Autodesk Inventor part; units mm, degrees
ref_plane "part2_to_part1_XY" through (0, 0, 0) normal (1, 0, 0) x (0, 0, -1)
ref_plane "part2_to_part1_YZ" through (0, 0, 0) normal (0, 0, -1) x (0, 1, 0)
ref_plane "part2_to_part1_ZX" through (0, 0, 0) normal (0, 1, 0) x (1, 0, 0)
sketch "Sketch_1" plane through (0, 0, 0) normal (0, 0, 1) x (1, 0, 0)
  line L0 (10, 0) -> (0, 0)
  line L1 (1, 5) -> (10, 5)
  line L2 (10, 5) -> (10, 12)
  line L3 (10, 12) -> (9.5, 12.5)
  line L4 (9.5, 12.5) -> (1, 12.5)
  line L5 (1, 12.5) -> (1, 5)
revolve "Revolution1" add sketch "Sketch_1" angle 180 mid plane about axis through (10, 0, 0) along (-1, 0, 0)
sketch "Sketch_2" plane through (0, 0, 0) normal (0, 0, 1) x (1, 0, 0)
  line L0 (0, 0.5) -> (0, 0)
  line L1 (0, 0) -> (20, 0)
  line L2 (20, 0) -> (20, 0.5)
  line L3 (20, 0.5) -> (0, 0.5)
extrude "Extrusion1" cut sketch "Sketch_2" along normal mid plane 50
sketch "Sketch_3" plane through (0, 0, 9) normal (0, 0, 1) x (1, 0, 0)
  line L0 (5.5, 12.5) -> (5.5, 0)
  line L1 (5.5, 0) -> (3.25, 0)
  line L2 (3.25, 0) -> (3.25, 4.5)
  line L3 (3.25, 4.5) -> (1.5, 4.5)
  line L4 (1.5, 4.5) -> (1.5, 12.5)
  line L5 (1.5, 12.5) -> (5.5, 12.5)
  line L6 (5.5, 12.5) -> (5.5, 0)
revolve "Revolution2" cut sketch "Sketch_3" angle 360 about axis through (5.5, 12.5, 9) along (0, 1, 0)
sketch "Sketch_4" plane through (0, 0, -9) normal (0, 0, 1) x (1, 0, 0)
  line L0 (5.5, 12.5) -> (5.5, 0)
  line L1 (5.5, 0) -> (3.25, 0)
  line L2 (3.25, 0) -> (3.25, 4.5)
  line L3 (3.25, 4.5) -> (1.5, 4.5)
  line L4 (1.5, 4.5) -> (1.5, 12.5)
  line L5 (1.5, 12.5) -> (5.5, 12.5)
  line L6 (5.5, 12.5) -> (5.5, 0)
revolve "Revolution3" cut sketch "Sketch_4" angle 360 about axis through (5.5, 12.5, -9) along (0, 1, 0)
sketch "Sketch_5" plane through (0, 0, 9) normal (0, 0, 1) x (1, 0, 0)
  line L0 (0, 17) -> (0, 4.5)
  line L1 (0, 4.5) -> (20, 4.5)
  line L2 (20, 4.5) -> (20, 17)
  line L3 (20, 17) -> (0, 17)
extrude "Extrusion2" cut sketch "Sketch_5" along normal blind 25
sketch "Sketch_6" plane through (0, 0, -9) normal (0, 0, 1) x (1, 0, 0)
  line L0 (0, 17) -> (0, 4.5)
  line L1 (0, 4.5) -> (20, 4.5)
  line L2 (20, 4.5) -> (20, 17)
  line L3 (20, 17) -> (0, 17)
extrude "Extrusion3" cut sketch "Sketch_6" against normal blind 25
ref_plane "part2_to_part1_XY" through (0, 0, 0) normal (1, 0, 0) x (0, 0, -1)
ref_plane "part2_to_part1_YZ" through (0, 0, 0) normal (0, 0, -1) x (0, 1, 0)
ref_plane "part2_to_part1_ZX" through (0, 0, 0) normal (0, 1, 0) x (1, 0, 0)
ref_plane "part2_to_screw1_XY" through (5.5, 4.5, 9) normal (0, 1, 0) x (1, 0, 0)
ref_plane "part2_to_screw1_YZ" through (5.5, 4.5, 9) normal (1, 0, 0) x (0, 0, -1)
ref_plane "part2_to_screw1_ZX" through (5.5, 4.5, 9) normal (0, 0, -1) x (0, 1, 0)
ref_plane "part2_to_screw2_XY" through (5.5, 4.5, -9) normal (0, 1, 0) x (1, 0, 0)
ref_plane "part2_to_screw2_YZ" through (5.5, 4.5, -9) normal (1, 0, 0) x (0, 0, -1)
ref_plane "part2_to_screw2_ZX" through (5.5, 4.5, -9) normal (0, 0, -1) x (0, 1, 0)
properties part number "MBRAC45-2-10p2"
CAD build for the part. Positions are in the model's coordinates, mm. A direction names the side the tool comes from. Coordinates: 2 decimals unless noted, no trailing zeros. Loops run counter-clockwise (first coordinate to the right, second up) from the corner with the lowest first, then second, coordinate; pieces in that order, holes last. Notation, with made-up numbers: (2, 70) - (14, 70) arc R18 cw to (14, 74) - close; hole circle Ø6 at (67.25, 37). An arc over 180 degrees is marked (long way). Use CSV: the item, a comma, the result in double quotes. Start each with the question number.
Q1. Cut at A-A, the plane x = 5.5. List the corners of the cut face in (y, z).
Q2. Probe probe 1 along X at (y, z) = (3.4, -9); probe 2 along Z at (x, y) = (5.5, 3.2); probe 3 along Z at (x, y) = (4.25, 1.25). List the from-to ranges inside material, lowest first. Write a range as from..to.
Q3. Cut at C-C, the plane y = 1.75. State how many separate pieces and enclosed holes the cut face has, then the cut area to 3 significant figures.
Q4. 3-axis set-ups, long thin cutter, end or side, ignore diameter. For faces 1 (the flat face through (7, 0.5, 7)), 2 (the flat face through (4, 4.5, 7)), 3 (the cylindrical face through (5.4, 7.3, -5)): which of +Z, -Z, +X, -X, +Y, -Y reach the whole face in a straight line?
Q5. Drop flat-ended pins along their axis: P1, Ø3.5, axis at x = 3.5, z = -9.5, coming from the +Y side; P2, Ø0.6, axis at x = 1, y = 6, coming from the +Z side; P3, Ø1, axis at x = 5, y = 3.5, coming from the +Z side. Give the stop position or say it passes through.
Q6. Cut at D-D, the plane x = 3.5. List the corners of the cut face in (y, z).
Q7. Cut at B-B, the plane y = 6.25. List the corners of the cut face in (x, z).
Q8. Two-plate mould, pull along X, no slides. Class faces 4 (the flat face through (4, 4.5, -7)), 5 (the flat face through (1, 7, 0)), 6 (the flat face through (8, 0.5, -8)), 7 (the cylindrical face through (4.29, 2.528, 10.897)): +X half, -X half, draft (parallel to the pull), parting line (faces both ways), or undercut.
Here are the results:
1,outline,"(0.5, -12.49) arc R12.5 ccw to (4.5, -11.66) - (4.5, -11.25) - (0.5, -11.25) - close; (0.5, -6.75) - (4.5, -6.75) - (4.5, -5) - (11.46, -5) arc R12.5 ccw to (11.46, 5) - (4.5, 5) - (4.5, 6.75) - (0.5, 6.75) - (0.5, 4.97) arc R5 cw to (0.5, -4.97) - close; (0.5, 11.25) - (4.5, 11.25) - (4.5, 11.66) arc R12.5 ccw to (0.5, 12.49) - close"
2,probe 1,"1..3.25, 7.75..10"
2,probe 2,"-12.08..-11.25, -6.75..-3.84, 3.84..6.75, 11.25..12.08"
2,probe 3,"-12.44..-10.87, -7.13..-4.84, 4.84..7.13, 10.87..12.44"
3,separate pieces,"2"
3,enclosed holes,"2"
3,area,"106 mm2"
4,face 1,"+Z, -Z, +X, -X, -Y"
4,face 2,"+Z, +Y"
4,face 3,"-Z, +Y"
5,P1,"y = 4.5"
5,P2,"z = 9"
5,P3,"z = 12.13"
6,outline,"(0.5, -12.49) arc R12.5 ccw to (4.5, -11.66) - (4.5, -10.03) - (0.5, -10.03) - close; (0.5, -7.97) - (4.5, -7.97) - (4.5, -5.54) - (11.21, -5.54) arc R12.5 ccw to (11.21, 5.54) - (4.5, 5.54) - (4.5, 7.97) - (0.5, 7.97) - (0.5, 4.97) arc R5 cw to (0.5, -4.97) - close; (0.5, 10.03) - (4.5, 10.03) - (4.5, 11.66) arc R12.5 ccw to (0.5, 12.49) - close"
7,outline,"(1, -9) - (1.5, -9) arc R4 cw to (9.5, -9) - (10, -9) - (10, 9) - (9.5, 9) arc R4 cw to (1.5, 9) - (1, 9) - close"
8,face 4,"undercut"
8,face 5,"-X half"
8,face 6,"draft"
8,face 7,"undercut"
